Read the model definition and answer for the solid it produces. Units are mm, in the model's axes. A direction names the side the tool comes from. Coordinates: 2 decimals unless noted, no trailing zeros. Write each loop counter-clockwise with the first axis right and the second up, starting at its lowest first coordinate (ties: lowest second). Pieces come first, ordered by that corner, then holes. Notation, with made-up numbers: (25.5, 31.5) -> (53.5, 31.5) arc R20 cw to (53.5, 61.5) -> close; hole circle Ø10 at (-2, 16). An arc over 180 degrees is marked (long way). Write item = value, one per line. Start each with the question number.
1) Section B-B (x = 0) is taken. Determine the outline of the cut face in (y, z), plus the area to 3 significant figures.
2) Section C-C (y = 2.75) is taken. Determine the outline of the cut face in (x, z), plus the area to 3 significant figures.
3) Find the intervals of material crossed by line 1 along X through (y, z) = (3.25, 0); line 2 along Z through (x, y) = (22, 2.55); line 3 along Z through (x, y) = (-0.5, 3.65), in increasing order. Write a range as from..to.
4) Section D-D (x = -22) is taken. Determine the outline of the cut face in (y, z), plus the area to 3 significant figures.
5) A flat-ended cylindrical pin translates along its axis: pin 1 Ø7 at (x, z) = (0, -7.5) entering from +Y. Find the tip coordinate at first contact, or state that the pin passes through.
6) For a pull along X with two mould halves and no side action, classify faces 1 (the face through (-32.5, 2, 0)), 2 (the face through (32.5, 2, 0)), 3 (the face through (0, 2, -12.5)), 4 (the face through (1.352, 0.986, -11.792)) as released by +X, released by -X, zero draft, split by the parting line, or undercut.
7) Section A-A (z = -7.5) is taken. Determine the outline of the cut face in (x, y).
8) A tool of negligible diameter and unlimited length cuts with its end or side. For faces 5 (the face through (-1.9, 2, -9.4)), 6 (the face through (18.034, 1.972, -0.521)), from which of +Z, -Z, +X, -X, +Y, -Y can it reach the whole face along a straight path? Write none if from no direction.
from build123d import *

# Parameters (mm, degrees)
SKETCH_1_W          = 65
SKETCH_1_H          = 25
EXTRUDE_1_DEPTH     = 4
SKETCH_2_W          = 15
SKETCH_2_H          = 25
EXTRUDE_2_DEPTH     = 13
SKETCH_3_R          = 2.5
SKETCH_3_R_2        = 4
CUT_EXTRUDE_1_DEPTH = 39.74919354
SKETCH_4_R          = 4.5
CUT_EXTRUDE_2_DEPTH = 2
SKETCH_5_W          = 15
SKETCH_5_H          = 4
EXTRUDE_3_DEPTH     = 6
SKETCH_6_R          = 1.25
CUT_EXTRUDE_3_DEPTH = 40.59166579
FILLET_2_R          = 3
SKETCH_9_W          = 15
SKETCH_9_H          = 13
CUT_EXTRUDE_4_DEPTH = 53.098464469


with BuildPart() as part:
    # 草图1 → 凸台-拉伸1 (new body)
    with BuildSketch(Plane(origin=(0, 0, 0), x_dir=(1, 0, 0), z_dir=(0, 1, 0))):
        Rectangle(SKETCH_1_W, SKETCH_1_H)
    extrude(amount=EXTRUDE_1_DEPTH)

    # 草图2 → 凸台-拉伸2 (add)
    with BuildSketch(Plane(origin=(0, 4, 0), x_dir=(1, 0, 0), z_dir=(0, 1, 0))):
        Rectangle(SKETCH_2_W, SKETCH_2_H)
    extrude(amount=EXTRUDE_2_DEPTH)

    # 草图3 → 切除-拉伸1 (cut, through all)
    with BuildSketch(Plane.XZ):
        with Locations(Location((0, -7.5, 0), (0, 0, 270))):
            Circle(SKETCH_3_R)
        with Locations(Location((0, 7.5, 0), (0, 0, 90))):
            Circle(SKETCH_3_R)
        with Locations(Location((-22, 0, 0), (0, 0, 270))):
            Circle(SKETCH_3_R_2)
        with Locations(Location((22, 0, 0), (0, 0, 90))):
            Circle(SKETCH_3_R_2)
    extrude(amount=-CUT_EXTRUDE_1_DEPTH, mode=Mode.SUBTRACT)

    # 草图4 → 切除-拉伸2 (cut)
    with BuildSketch(Plane.XZ):
        with Locations(Location((0, -7.5, 0), (0, 0, 270))):
            Circle(SKETCH_4_R)
        with Locations(Location((0, 7.5, 0), (0, 0, 270))):
            Circle(SKETCH_4_R)
    extrude(amount=-CUT_EXTRUDE_2_DEPTH, mode=Mode.SUBTRACT)

    # 草图5 → 凸台-拉伸3 (add)
    with BuildSketch(Plane.XY.offset(12.5)):
        with Locations((0, 6)):
            Rectangle(SKETCH_5_W, SKETCH_5_H)
    extrude_3 = extrude(amount=EXTRUDE_3_DEPTH)

    # 草图6 → 切除-拉伸3 (cut, through all)
    with BuildSketch(Plane.XZ.offset(-4)):
        with Locations(Location((-4.5, 15.5, 0), (0, 0, 270))):
            Circle(SKETCH_6_R)
        with Locations(Location((4.5, 15.5, 0), (0, 0, 270))):
            Circle(SKETCH_6_R)
    cut_extrude_3 = extrude(amount=-CUT_EXTRUDE_3_DEPTH, mode=Mode.SUBTRACT)

    # 镜向2: 凸台-拉伸3, 切除-拉伸3 across plane
    add(extrude_3.mirror(Plane.XY))
    add(cut_extrude_3.mirror(Plane.XY), mode=Mode.SUBTRACT)

    # 圆角2
    fillet_2_edges = [part.edges().sort_by_distance(p)[0] for p in [
        (-7.5, 6, 18.5),
        (7.5, 6, 18.5),
        (-7.5, 6, -18.5),
        (7.5, 6, -18.5),
    ]]
    fillet(fillet_2_edges, radius=FILLET_2_R)

    # 草图9 → 切除-拉伸4 (cut, through all)
    with BuildSketch(Plane.XY.offset(18.5)):
        with Locations((0, 10.5)):
            Rectangle(SKETCH_9_W, SKETCH_9_H)
    extrude(amount=-CUT_EXTRUDE_4_DEPTH, mode=Mode.SUBTRACT)


solid = part.part
Answer key:
q1.outline = (0, -12.5) -> (4, -12.5) -> (4, -10) -> (2, -10) -> (2, -12) -> (0, -12) -> close; (0, -3) -> (2, -3) -> (2, -5) -> (4, -5) -> (4, 5) -> (2, 5) -> (2, 3) -> (0, 3) -> close; (0, 12) -> (2, 12) -> (2, 10) -> (4, 10) -> (4, 12.5) -> (0, 12.5) -> close
q1.area = 44.0 mm^2
q2.outline = (-32.5, -12.5) -> (32.5, -12.5) -> (32.5, 12.5) -> (-32.5, 12.5) -> close; hole circle Ø8 at (-22, 0); hole circle Ø5 at (0, -7.5); hole circle Ø5 at (0, 7.5); hole circle Ø8 at (22, 0)
q2.area = 1,490 mm^2
q3.line_1 = -32.5..-26, -18..18, 26..32.5
q3.line_2 = -12.5..-4, 4..12.5
q3.line_3 = -12.5..-9.95, -5.05..5.05, 9.95..12.5
q4.outline = (0, -12.5) -> (4, -12.5) -> (4, -4) -> (0, -4) -> close; (0, 4) -> (4, 4) -> (4, 12.5) -> (0, 12.5) -> close
q4.area = 68.0 mm^2
q5.pin_1 = 4
q6.face_1 = released by -X
q6.face_2 = released by +X
q6.face_3 = zero draft
q6.face_4 = undercut
q7.outline = (-32.5, 0) -> (-4.5, 0) -> (-4.5, 2) -> (-2.5, 2) -> (-2.5, 4) -> (-32.5, 4) -> close; (2.5, 2) -> (4.5, 2) -> (4.5, 0) -> (32.5, 0) -> (32.5, 4) -> (2.5, 4) -> close
q8.face_5 = -Y
q8.face_6 = +Y, -Y
